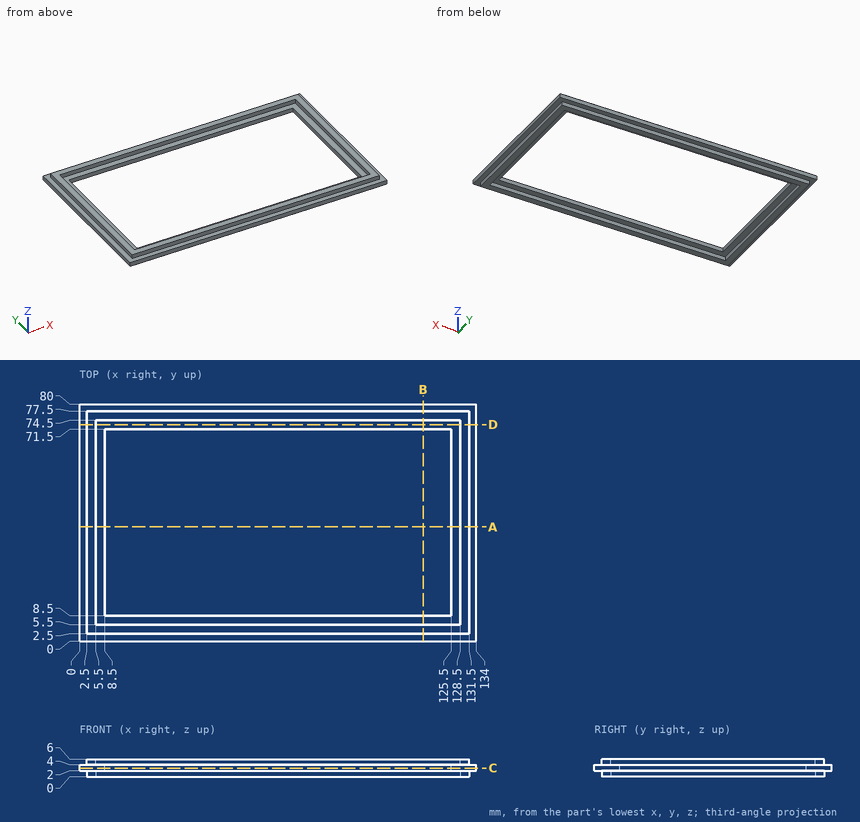
Could you check a few things on this drawing? It's one solid part, dimensions in mm from its lowest x, y, z. Give positions to 0.01 mm unless a question says otherwise; leave off trailing zeros. Order: outer loops, then holes, each group sorted by start corner. A loop starts at its lowest first (then second) coordinate and runs counter-clockwise, first axis right, second up. Notation, with made-up numbers: M -36.75,61.25 L -28.75,61.25 A24 cw -28.75,90.25 Z; hole C 26,72.25 d8. An arc over 180 degrees is marked long. Use one line per item in the form item = value.
Item 1: If we section it at D-D, the plane y = 73: Write out the boundary of the cut face in (x, z), and give its area (3 significant figures).
Values follow:
outline = M 0,2 L 2.5,2 L 2.5,0 L 5.5,0 L 5.5,2 L 128.5,2 L 128.5,0 L 131.5,0 L 131.5,2 L 134,2 L 134,4 L 131.5,4 L 131.5,6 L 128.5,6 L 128.5,4 L 5.5,4 L 5.5,6 L 2.5,6 L 2.5,4 L 0,4 Z
area = 292 mm^2
Item 2: Will these pins go through, and if not, where does the flat tip stop? pin 1 Ø1.5 at (y, z) = (59, 1) entering from +X; pin 2 Ø6 at (x, y) = (120.5, 39) entering from +Z; pin 3 Ø6 at (x, y) = (53, 69.5) entering from -Z; pin 4 Ø1 at (x, z) = (78, 5.5) entering from -Y.
Values follow:
pin_1 = 131.5
pin_2 = through
pin_3 = 2
pin_4 = 2.5
Item 3: If we section it at B-B, the plane x = 116: Write out the boundary of the cut face in (y, z).
Values follow:
outline = M 0,2 L 2.5,2 L 2.5,0 L 5.5,0 L 5.5,2 L 8.5,2 L 8.5,4 L 5.5,4 L 5.5,6 L 2.5,6 L 2.5,4 L 0,4 Z; M 71.5,2 L 74.5,2 L 74.5,0 L 77.5,0 L 77.5,2 L 80,2 L 80,4 L 77.5,4 L 77.5,6 L 74.5,6 L 74.5,4 L 71.5,4 Z
Item 4: If we section it at C-C, the plane z = 2.9: Write out the boundary of the cut face in (x, y).
Values follow:
outline = M 0,0 L 134,0 L 134,80 L 0,80 Z; hole M 8.5,8.5 L 125.5,8.5 L 125.5,71.5 L 8.5,71.5 Z
Item 5: If we section it at A-A, the plane y = 38.5: Write out the boundary of the cut face in (x, z), and give its area (3 significant figures).
Values follow:
outline = M 0,2 L 2.5,2 L 2.5,0 L 5.5,0 L 5.5,2 L 8.5,2 L 8.5,4 L 5.5,4 L 5.5,6 L 2.5,6 L 2.5,4 L 0,4 Z; M 125.5,2 L 128.5,2 L 128.5,0 L 131.5,0 L 131.5,2 L 134,2 L 134,4 L 131.5,4 L 131.5,6 L 128.5,6 L 128.5,4 L 125.5,4 Z
area = 58.0 mm^2
Item 6: If I drill on line 1 along Y through (x, z) = (15.5, 0.8); line 2 along X through (y, z) = (51.5, 5.4); line 3 along Y through (x, z) = (113, 2.65), over which ranges is the centre line in solid material (lowest first)? Write a range as [from, to].
Values follow:
line_1 = [2.5, 5.5], [74.5, 77.5]
line_2 = [2.5, 5.5], [128.5, 131.5]
line_3 = [0, 8.5], [71.5, 80]
